from build123d import *

# Parameters (mm, degrees)
BASPROSKE_W          = 10
BASPROSKE_H          = 12
TOOTHCUT_DEPTH       = 20.697715604
TEETHCUTS_COUNT      = 22
TEETHCUTS_ANGLE      = 343.636363636
BORSKE_R             = 5
BORE_DEPTH           = 50.0000508
D_GAGEMENT_M21_D     = 2
D_GAGEMENT_M21_DEPTH = 10


with BuildPart() as part:
    # BasProSke → Base-Revolve (revolve)
    with BuildSketch(Plane(origin=(0, 0, 0), x_dir=(1, 0, 0), z_dir=(0, 1, 0)), mode=Mode.PRIVATE) as base_revolve_sk:
        with Locations((5, 6)):
            Rectangle(BASPROSKE_W, BASPROSKE_H)
    revolve(base_revolve_sk.sketch.rotate(Axis((-10, 0, 0), (1, 0, 0)), 180), axis=Axis((-10, 0, 0), (1, 0, 0)))

    # TooCutSke → ToothCut (cut, through all)
    with BuildSketch(Plane(origin=(0, 0, 0), x_dir=(0, 0, -1), z_dir=(1, 0, 0))):
        with BuildLine():
            ThreePointArc((0.491001901, 9.736627657), (0, 9.749), (-0.491001901, 9.736627657))
            ThreePointArc((-0.491001901, 9.736627657), (-0.822824844, 10.904005344), (-1.46093845, 11.936327074))
            ThreePointArc((-1.46093845, 11.936327074), (0, 12.0254), (1.46093845, 11.936327074))
            ThreePointArc((1.46093845, 11.936327074), (0.822824844, 10.904005344), (0.491001901, 9.736627657))
        make_face()
    toothcut = extrude(amount=TOOTHCUT_DEPTH, mode=Mode.SUBTRACT)

    # TeethCuts: ToothCut ×22 about axis
    teethcuts_axis = Axis((-10, 0, 0), (1, 0, 0))
    for i in range(1, TEETHCUTS_COUNT):
        add(toothcut.rotate(teethcuts_axis, i * TEETHCUTS_ANGLE / (TEETHCUTS_COUNT - 1)), mode=Mode.SUBTRACT)

    # BorSke → Bore (cut, symmetric)
    with BuildSketch(Plane(origin=(0, 0, 0), x_dir=(0, 0, -1), z_dir=(1, 0, 0))):
        with Locations(Location((0, 0, 0), (0, 0, 180))):
            Circle(BORSKE_R)
    extrude(amount=BORE_DEPTH, both=True, mode=Mode.SUBTRACT)

    # Dégagement M21
    with Locations(Plane(origin=(10, 0, 0), x_dir=(0, 0, -1), z_dir=(1, 0, 0))):
        with Locations((0, 7), (4.949747468, 4.949747468), (7, 0), (4.949747468, -4.949747468), (0, -7), (-4.949747468, -4.949747468), (-7, 0), (-4.949747468, 4.949747468), (0, 0)):
            Hole(D_GAGEMENT_M21_D / 2, depth=D_GAGEMENT_M21_DEPTH)


solid = part.part
Input: part model. Units: mm. Frame: model coordinates. A direction names the side the tool comes from. Coordinates: 2 decimals unless noted, no trailing zeros. Loops run counter-clockwise (first coordinate to the right, second up) from the corner with the lowest first, then second, coordinate; pieces in that order, holes last.
(1) Material intervals for probe 1 along Y at (x, z) = (3, -9); probe 2 along Z at (x, y) = (9, -5.25); probe 3 along Y at (x, z) = (5, 10), sorted ascending.
(2) Section B-B on y = -7.5. Return the cut outline in (x, z), then the cut area to 3 significant figures.
(3) Section C-C on x = 2.5. Count the separate pieces of the cut face and the enclosed holes in it, then the cut area to 3 significant figures.
(4) Section A-A on z = 0. Return the cut outline in (x, y).
(5) Set-up query: faces 1 (the face through (4.93, 10.206, 3.841)), 2 (the face through (4.93, -8.73, 6.59)), 3 (the face through (4.93, -6.51, -8.75)). Return all of +Z, -Z, +X, -X, +Y, -Y with unobstructed straight access to the full face (end or side cutting, diameter ignored); none if empty.
(6) Pull-direction query (Z, two-part tool) for faces 4 (the face through (4.93, -1.39, -9.65)), 5 (the face through (4.93, 1.39, 9.65)), 6 (the face through (4.93, 10.7, 2.28)); classes: released by +Z, released by -Z, zero draft, split by the parting line, or undercut.
(7) Section D-D on y = -2.75. Return the cut outline in (x, z), then the cut area to 3 significant figures.
(8) First-contact query: pin 1 Ø4 at (x, y) = (4, 3) entering from +Z; pin 2 Ø1 at (x, y) = (5, -2.5) entering from -Z. Flat tips, straight axial feed; report the tip coordinate or a pass-through.
Data:
1. probe 1: y = -6.58 to -4.74, -3.75 to 3.75, 4.74 to 6.58
1. probe 2: z = -9.55 to -5.9, -4 to 4, 5.9 to 9.55
1. probe 3: y = -6.63 to -5.84, -3.77 to -2.02, -0.89 to 0.89, 2.02 to 3.77, 5.84 to 6.63
2. outline: (0, -7.57) - (10, -7.57) - (10, -0.87) - (0, -0.87) - close; (0, 0.87) - (10, 0.87) - (10, 7.57) - (0, 7.57) - close
2. area: 134 mm2
3. separate pieces: 1
3. enclosed holes: 9
3. area: 264 mm2
4. outline: (0, -9.75) - (10, -9.75) - (10, -8) - (0, -8) - close; (0, -6) - (10, -6) - (10, -5) - (0, -5) - close; (0, 5) - (10, 5) - (10, 6) - (0, 6) - close; (0, 8) - (10, 8) - (10, 9.75) - (0, 9.75) - close
5. face 1: +X, -X, +Y
5. face 2: +X, -X, -Y
5. face 3: +X, -X
6. face 4: released by -Z
6. face 5: released by +Z
6. face 6: undercut
7. outline: (0, -11.2) - (10, -11.2) - (10, -4.18) - (0, -4.18) - close; (0, 4.18) - (10, 4.18) - (10, 11.2) - (0, 11.2) - close
7. area: 140 mm2
8. pin 1: stops at z = 11.59
8. pin 2: stops at z = -11.47
